For this review, take the finished solid that the model builds, in its own axes (mm). Coordinates: 2 decimals unless noted, no trailing zeros. Loops run counter-clockwise (first coordinate to the right, second up) from the corner with the lowest first, then second, coordinate; pieces in that order, holes last. Notation, with made-up numbers: M 38,-10 L 82,-10 A18 ccw 82,-6 Z; hole C -29.5,1 d10. An arc over 180 degrees is marked long. Answer as a JSON object with one key per item and string values. Group by question number.
Item 1: Wall thickness on L1, parallel to X at y = 1.2, z = -0.8; L2, parallel to Z at x = -2.5, y = 1.1; L3, parallel to Y at x = 6.75, z = -1.05: over which ranges is each line inside the solid? List them lowest first. Write a range as from..to.
Item 2: Insertion check: pin 1 (0.5 mm diameter, centred on x = 4, z = -1, fed in from +Y); pin 2 (0.5 mm diameter, centred on x = -0.5, z = -1, fed in from -Y); pin 3 (1.3 mm diameter, centred on y = 2.5, z = -1, fed in from -X). Each pin has a flat end and moves straight along its axis. Give the tip position at first contact, or say it passes through.
Item 3: Add section A-A (x = 1.25). State the section outline as (y, z) points, then the cut area to 3 significant figures.
Item 4: Add section B-B (y = 2.75). State the section outline as (x, z) points, then the cut area to 3 significant figures.
Item 5: Add section C-C (z = -0.45). State the section outline as (x, y) points.
from build123d import *

# Parameters (mm, degrees)
SKETCH1_W               = 2.54
SKETCH1_H               = 2.54
BOSS_EXTRUDE1_DEPTH     = 3.56
SKETCH2_W               = 0.64
SKETCH2_H               = 0.64
BOSS_EXTRUDE2_DEPTH     = 5.84
CHAMFER1_SIZE           = 0.57
CHAMFER2_SIZE           = 1
CHAMFER2_SIZE2          = 0.176326981
CHAMFER2_PART_2_SIZE    = 1
CHAMFER2_PART_2_SIZE2   = 0.176326981
CHAMFER2_PART_3_SIZE    = 1
CHAMFER2_PART_3_SIZE2   = 0.176326981
CHAMFER2_PART_4_SIZE    = 1
CHAMFER2_PART_4_SIZE2   = 0.176326981
SKETCH3_W               = 0.64
SKETCH3_H               = 0.64
BOSS_EXTRUDE3_DEPTH     = 2.285
SKETCH4_W               = 0.64
SKETCH4_H               = 0.64
BOSS_EXTRUDE4_DEPTH     = 2.285
CHAMFER3_SIZE           = 1
CHAMFER3_SIZE2          = 0.176326981
CHAMFER3_PART_2_SIZE    = 1
CHAMFER3_PART_2_SIZE2   = 0.176326981
CHAMFER3_PART_3_SIZE    = 1
CHAMFER3_PART_3_SIZE2   = 0.176326981
CHAMFER3_PART_4_SIZE    = 1
CHAMFER3_PART_4_SIZE2   = 0.176326981
BOSS_EXTRUDE5_DEPTH     = 0.64
CUT_EXTRUDE1_DEPTH      = 1.95
CUT_EXTRUDE1_DEPTH_BACK = 2.59


with BuildPart() as part:
    # Sketch1 → Boss-Extrude1 (new body)
    with BuildSketch(Plane(origin=(0, 0, 0), x_dir=(1, 0, 0), z_dir=(0, 1, 0))):
        with Locations((1.27, 1.27)):
            Rectangle(SKETCH1_W, SKETCH1_H)
    extrude(amount=BOSS_EXTRUDE1_DEPTH)

    # Sketch2 → Boss-Extrude2 (add)
    with BuildSketch(Plane(origin=(2.54, 0, 0), x_dir=(0, 0, -1), z_dir=(1, 0, 0))):
        with Locations((1.27, 1.78)):
            Rectangle(SKETCH2_W, SKETCH2_H)
    extrude(amount=BOSS_EXTRUDE2_DEPTH)

    # Chamfer1
    chamfer1_edges = [part.edges().sort_by_distance(p)[0] for p in [
        (1.27, 3.56, -2.54),
        (1.27, 0, -2.54),
        (1.27, 0, 0),
        (1.27, 3.56, 0),
    ]]
    chamfer(chamfer1_edges, length=CHAMFER1_SIZE)

    # Chamfer2
    chamfer2_edges = [part.edges().sort_by_distance(p)[0] for p in [
        (8.38, 1.78, -0.95),
    ]]
    chamfer2_side = [part.faces().sort_by_distance(p)[0] for p in [
        (5.46, 1.78, -0.95),
    ]]
    chamfer(chamfer2_edges, length=CHAMFER2_SIZE, length2=CHAMFER2_SIZE2, reference=chamfer2_side[0])

    # Chamfer2 part 2
    chamfer2_part_2_edges = [part.edges().sort_by_distance(p)[0] for p in [
        (8.38, 1.46, -1.27),
    ]]
    chamfer2_part_2_side = [part.faces().sort_by_distance(p)[0] for p in [
        (5.46, 1.46, -1.27),
    ]]
    chamfer(chamfer2_part_2_edges, length=CHAMFER2_PART_2_SIZE, length2=CHAMFER2_PART_2_SIZE2, reference=chamfer2_part_2_side[0])

    # Chamfer2 part 3
    chamfer2_part_3_edges = [part.edges().sort_by_distance(p)[0] for p in [
        (8.38, 1.78, -1.59),
    ]]
    chamfer2_part_3_side = [part.faces().sort_by_distance(p)[0] for p in [
        (5.46, 1.78, -1.59),
    ]]
    chamfer(chamfer2_part_3_edges, length=CHAMFER2_PART_3_SIZE, length2=CHAMFER2_PART_3_SIZE2, reference=chamfer2_part_3_side[0])

    # Chamfer2 part 4
    chamfer2_part_4_edges = [part.edges().sort_by_distance(p)[0] for p in [
        (8.38, 2.1, -1.27),
    ]]
    chamfer2_part_4_side = [part.faces().sort_by_distance(p)[0] for p in [
        (5.46, 2.1, -1.27),
    ]]
    chamfer(chamfer2_part_4_edges, length=CHAMFER2_PART_4_SIZE, length2=CHAMFER2_PART_4_SIZE2, reference=chamfer2_part_4_side[0])

    # Sketch3 → Boss-Extrude3 (add)
    with BuildSketch(Plane.ZY):
        with Locations((-1.27, 1.78)):
            Rectangle(SKETCH3_W, SKETCH3_H)
    extrude(amount=BOSS_EXTRUDE3_DEPTH)



with BuildPart() as body_2:
    # Sketch4 → Boss-Extrude4 (new body)
    with BuildSketch(Plane.ZY.offset(2.285)):
        with Locations((-1.27, 0.32)):
            Rectangle(SKETCH4_W, SKETCH4_H)
    extrude(amount=BOSS_EXTRUDE4_DEPTH)

    # Chamfer3
    chamfer3_edges = [body_2.edges().sort_by_distance(p)[0] for p in [
        (-4.57, 0.32, -1.59),
    ]]
    chamfer3_side = [body_2.faces().sort_by_distance(p)[0] for p in [
        (-3.4275, 0.32, -1.59),
    ]]
    chamfer(chamfer3_edges, length=CHAMFER3_SIZE, length2=CHAMFER3_SIZE2, reference=chamfer3_side[0])

    # Chamfer3 part 2
    chamfer3_part_2_edges = [body_2.edges().sort_by_distance(p)[0] for p in [
        (-4.57, 0, -1.27),
    ]]
    chamfer3_part_2_side = [body_2.faces().sort_by_distance(p)[0] for p in [
        (-3.4275, 0, -1.27),
    ]]
    chamfer(chamfer3_part_2_edges, length=CHAMFER3_PART_2_SIZE, length2=CHAMFER3_PART_2_SIZE2, reference=chamfer3_part_2_side[0])

    # Chamfer3 part 3
    chamfer3_part_3_edges = [body_2.edges().sort_by_distance(p)[0] for p in [
        (-4.57, 0.32, -0.95),
    ]]
    chamfer3_part_3_side = [body_2.faces().sort_by_distance(p)[0] for p in [
        (-3.4275, 0.32, -0.95),
    ]]
    chamfer(chamfer3_part_3_edges, length=CHAMFER3_PART_3_SIZE, length2=CHAMFER3_PART_3_SIZE2, reference=chamfer3_part_3_side[0])

    # Chamfer3 part 4
    chamfer3_part_4_edges = [body_2.edges().sort_by_distance(p)[0] for p in [
        (-4.57, 0.64, -1.27),
    ]]
    chamfer3_part_4_side = [body_2.faces().sort_by_distance(p)[0] for p in [
        (-3.4275, 0.64, -1.27),
    ]]
    chamfer(chamfer3_part_4_edges, length=CHAMFER3_PART_4_SIZE, length2=CHAMFER3_PART_4_SIZE2, reference=chamfer3_part_4_side[0])


with BuildPart() as part_1:
    add(part.part)

    add(body_2.part)  # Boss-Extrude5 merges body 2
    # Sketch5 → Boss-Extrude5 (add)
    with BuildSketch(Plane(origin=(0, 0, -1.59), x_dir=(-1, 0, 0), z_dir=(0, 0, -1))):
        Polygon((2.285, 0.525518207), (1.1425, 1.46), (2.153367279, 1.46), (3.155901525, 0.64), (2.285, 0.64), align=None)
    extrude(amount=-BOSS_EXTRUDE5_DEPTH)

    # Sketch6 → Cut-Extrude1 (cut, two sides)
    with BuildSketch(Plane(origin=(0, 0, -1.59), x_dir=(-1, 0, 0), z_dir=(0, 0, -1))) as cut_extrude1_sk:
        Polygon((2.153367279, 1.46), (1.370901525, 2.1), (2.285, 2.1), (2.285, 1.46), align=None)
        Polygon((2.285, 0.525518207), (2.9275, 0), (2.285, 0), align=None)
    extrude(amount=CUT_EXTRUDE1_DEPTH, mode=Mode.SUBTRACT)
    extrude(cut_extrude1_sk.sketch, amount=-CUT_EXTRUDE1_DEPTH_BACK, mode=Mode.SUBTRACT)


solid = part_1.part
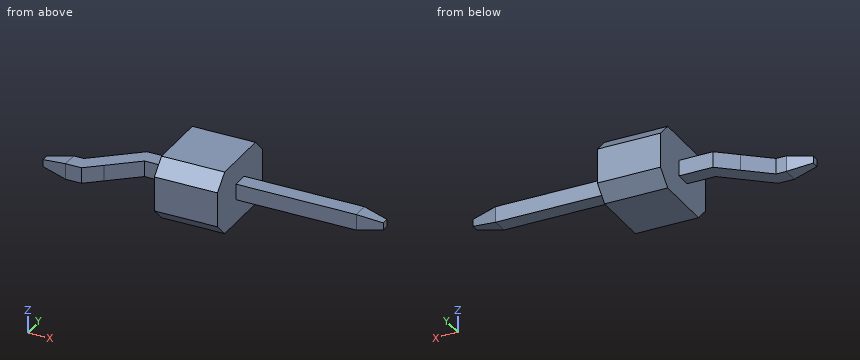
From the geometry:
{
 "1": {"L1": "x = 0..2.54", "L2": "z = -1.59..-0.95", "L3": "y = 1.46..2.1"},
 "2": {"pin 1": "stops at y = 2.1", "pin 2": "stops at y = 1.46", "pin 3": "stops at x = -1.68"},
 "3": {"outline": "M 0,-1.97 L 0.57,-2.54 L 2.99,-2.54 L 3.56,-1.97 L 3.56,-0.57 L 2.99,0 L 0.57,0 L 0,-0.57 Z", "area": "8.39 mm²"},
 "4": {"outline": "M 0,-2.54 L 2.54,-2.54 L 2.54,0 L 0,0 Z", "area": "6.45 mm²"},
 "5": {"outline": "M 0,0.12 L 2.54,0.12 L 2.54,3.44 L 0,3.44 Z"}
}
